Check sheet for the modelled part. Datum: model origin and axes. Units: mm. A direction names the side the tool comes from. Round coordinates to 2 decimals unless told otherwise and drop trailing zeros. Order: outer loops, then holes, each group sorted by start corner. A loop starts at its lowest first (then second) coordinate and runs counter-clockwise, first axis right, second up. Notation, with made-up numbers: M 55.5,70.25 L 99.5,70.25 A18 ccw 99.5,98.25 Z; hole C -20,-35.75 d9. An arc over 180 degrees is marked long. One line per item, written item: value. Start each with the question number.
(1) Depth check by flat-ended pin: pin 1 Ø2 at (y, z) = (2, 9.5) entering from -X; pin 2 Ø3 at (x, y) = (-2, -6) entering from -Z; pin 3 Ø5 at (x, z) = (5.5, 4) entering from -Y. Enter the tip coordinate at first touch or a pass-through.
(2) Access from +Z, -Z, +X, -X, +Y, -Y to the whole of each face (thin tool, end or side, straight path). Record for faces 4 (the face through (2, -1, -6)), 5 (the face through (0, 0, 0.5)), 6 (the face through (0, 0, -1)).
(3) Cross-section at A-A, the plane y = 0. Enter the section's corners in (x, z) (3 decimals), and give its area (3 significant figures).
(4) Thickness scan on L1, parallel to Y at x = 0, z = 6.25; L2, parallel to Y at x = 0, z = -4.1 (3 decimals); L3, parallel to Z at x = 5.25, y = -3.5. Record the ranges inside material, lowest first.
(5) Release check for a two-part mould opening along Y. For faces 1 (the face through (-4, -2, 0)), 2 (the face through (0, -2, -4)), 3 (the face through (0.86, -3.88, -2.96)) record: released by +Y, released by -Y, zero draft, split by the parting line, or undercut.
(6) Cross-section at C-C, the plane z = -2.25. Enter the section's corners in (x, y) (3 decimals).
(7) Cross-section at D-D, the plane y = 3.25. Enter the section's corners in (x, z), and give its area (3 significant figures).
from build123d import *

# Parameters (mm, degrees)
SKETCH1_R           = 8
BOSS_EXTRUDE1_DEPTH = 13.5
SKETCH3_R           = 3.975
BOSS_EXTRUDE2_DEPTH = 6
SKETCH4_R           = 2.5
CUT_EXTRUDE2_DEPTH  = 13
SKETCH7_R           = 2
CUT_EXTRUDE3_DEPTH  = 5


with BuildPart() as part:
    # Sketch1 → Boss-Extrude1 (new body)
    with BuildSketch(Plane.XY):
        Circle(SKETCH1_R)
    extrude(amount=BOSS_EXTRUDE1_DEPTH)

    # Sketch3 → Boss-Extrude2 (add)
    with BuildSketch(Plane(origin=(0, 0, 0), x_dir=(-1, 0, 0), z_dir=(0, 0, -1))):
        Circle(SKETCH3_R)
    extrude(amount=BOSS_EXTRUDE2_DEPTH)

    # Sketch4 → Cut-Extrude2 (cut)
    with BuildSketch(Plane.XY.offset(13.5)):
        Circle(SKETCH4_R)
    extrude(amount=-CUT_EXTRUDE2_DEPTH, mode=Mode.SUBTRACT)

    # Sketch7 → Cut-Extrude3 (cut)
    with BuildSketch(Plane(origin=(0, 0, -6), x_dir=(-1, 0, 0), z_dir=(0, 0, -1))):
        Circle(SKETCH7_R)
    extrude(amount=-CUT_EXTRUDE3_DEPTH, mode=Mode.SUBTRACT)


solid = part.part
Values found:
1. pin 1: x = -7.94
1. pin 2: z = 0
1. pin 3: y = -7.42
2. face 4: -Z, +X, -X, +Y, -Y
2. face 5: +Z
2. face 6: -Z
3. outline: M -8,0 L -3.975,0 L -3.975,-6 L -2,-6 L -2,-1 L 2,-1 L 2,-6 L 3.975,-6 L 3.975,0 L 8,0 L 8,13.5 L 2.5,13.5 L 2.5,0.5 L -2.5,0.5 L -2.5,13.5 L -8,13.5 Z
3. area: 179 mm^2
4. L1: -8 to -2.5, 2.5 to 8
4. L2: -3.975 to -2, 2 to 3.975
4. L3: 0 to 13.5
5. face 1: zero draft
5. face 2: undercut
5. face 3: split by the parting line
6. outline: C 0,0 d7.95; hole C 0,0 d4
7. outline: M -7.31,0 L -2.29,0 L -2.29,-6 L 2.29,-6 L 2.29,0 L 7.31,0 L 7.31,13.5 L -7.31,13.5 Z
7. area: 225 mm^2
